The model under review builds one solid part; all positions refer to its coordinate system, in mm. Coordinates: 2 decimals unless noted, no trailing zeros. Order: outer loops, then holes, each group sorted by start corner. A loop starts at its lowest first (then second) coordinate and runs counter-clockwise, first axis right, second up. Notation, with made-up numbers: (-27, 36) -> (-11, 36) arc R25 ccw to (-11, 64) -> close; hole circle Ø11 at (-15, 70.25). An arc over 180 degrees is marked (long way). Use one line per item in the form item = value. Start each with the question number.
(1) Wall thickness on line 1 along Y through (x, z) = (-1.5, 12.5); line 2 along Z through (x, y) = (-2.1, -142.24); line 3 along Y through (x, z) = (-1, 13.5): over which ranges is each line inside the solid? List them lowest first.
(2) Insertion check: pin 1 Ø4.5 at (x, y) = (-15, 19.5) entering from +Z; pin 2 Ø5 at (y, z) = (-142.24, 9.906) entering from -X; pin 3 Ø1 at (y, z) = (-92, 8.5) entering from -X. Each pin has a flat end and moves straight along its axis. Give the tip position at first contact, or say it passes through.
(3) Take a section at C-C (y = 78). State the section outline as (x, z) points, then the cut area to 3 significant figures.
(4) Take a section at D-D (z = 16.5). State the section outline as (x, y) points, then the cut area to 3 significant figures.
(5) Take a section at A-A (y = 142.24). State the section outline as (x, z) points.
(6) Take a section at B-B (x = -8.5). State the section outline as (y, z) points, then the cut area to 3 significant figures.
```python
from build123d import *

# Parameters (mm, degrees)
F1_DEPTH = 152.4
F3_D     = 7.9375
F3_DEPTH = 17.4625
F3_TIP   = 2.3846655818
F5_D     = 7.9375
F5_DEPTH = 17.4752
F5_TIP   = 2.3846655818


with BuildPart() as f1:
    # F0 (on Front) → F1 (new body, symmetric)
    with BuildSketch(Plane.XZ):
        Polygon((-19.05, 0), (0, 0), (0, 19.05), (-3.2512, 19.05), (-3.2512, 3.2512), (-19.05, 3.2512), align=None)
    extrude(amount=F1_DEPTH, both=True)

    # F3
    with Locations(Plane.XY.offset(3.2512)):
        with Locations((-9.906, -142.24), (-9.906, 142.24)):
            Hole(F3_D / 2, depth=F3_DEPTH)
            with Locations((0, 0, -(F3_DEPTH + F3_TIP / 2))):  # 118° drill point
                Cone(0, F3_D / 2, F3_TIP, mode=Mode.SUBTRACT)

    # F5
    with Locations(Plane(origin=(-3.2512, 0, 0), x_dir=(0, -1, 0), z_dir=(-1, 0, 0))):
        with Locations((-142.24, 9.906), (142.24, 9.906)):
            Hole(F5_D / 2, depth=F5_DEPTH)
            with Locations((0, 0, -(F5_DEPTH + F5_TIP / 2))):  # 118° drill point
                Cone(0, F5_D / 2, F5_TIP, mode=Mode.SUBTRACT)


solid = f1.part
```
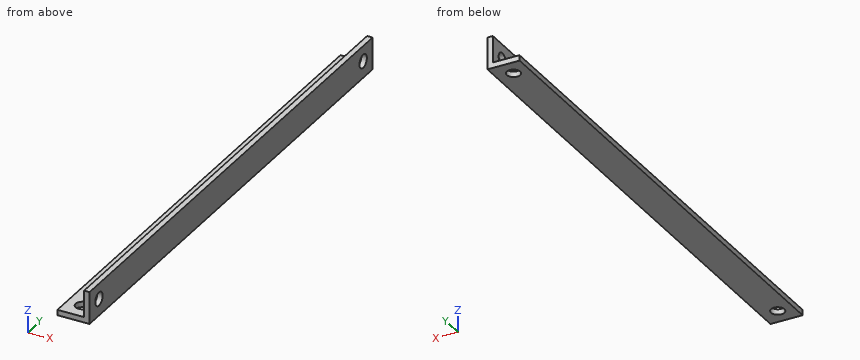
Findings:
q1.line_1 = -152.4 to -145.24, -139.24 to 139.24, 145.24 to 152.4
q1.line_2 = 0 to 5.94, 13.87 to 19.05
q1.line_3 = -152.4 to -143.92, -140.56 to 140.56, 143.92 to 152.4
q2.pin_1 = 3.25
q2.pin_2 = through
q2.pin_3 = -3.25
q3.outline = (-19.05, 0) -> (0, 0) -> (0, 19.05) -> (-3.25, 19.05) -> (-3.25, 3.25) -> (-19.05, 3.25) -> close
q3.area = 113 mm²
q4.outline = (-3.25, -152.4) -> (0, -152.4) -> (0, 152.4) -> (-3.25, 152.4) -> close
q4.area = 991 mm²
q5.outline = (-19.05, 0) -> (-13.87, 0) -> (-13.87, 3.25) -> (-19.05, 3.25) -> close; (-5.94, 0) -> (0, 0) -> (0, 5.94) -> (-3.25, 5.94) -> (-3.25, 3.25) -> (-5.94, 3.25) -> close; (-3.25, 13.87) -> (0, 13.87) -> (0, 19.05) -> (-3.25, 19.05) -> close
q6.outline = (-152.4, 0) -> (-145.95, 0) -> (-145.95, 3.25) -> (-152.4, 3.25) -> close; (-138.53, 0) -> (138.53, 0) -> (138.53, 3.25) -> (-138.53, 3.25) -> close; (145.95, 0) -> (152.4, 0) -> (152.4, 3.25) -> (145.95, 3.25) -> close
q6.area = 943 mm²
